Autodesk Inventor part; units mm, degrees
ref_plane "YZ Plane" through (0, 0, 0) normal (1, 0, 0) x (0, 1, 0)
ref_plane "XZ Plane" through (0, 0, 0) normal (0, 1, 0) x (-1, 0, 0)
ref_plane "XY Plane" through (0, 0, 0) normal (0, 0, 1) x (1, 0, 0)
sketch "Sketch1" plane through (0, 0, 0) normal (0, 1, 0) x (-1, 0, 0)
  line L0 (-25.4, 76.2) -> (25.4, 76.2)
  line L1 (50.8, 76.2) -> (-50.8, 76.2)
  line L2 (-50.8, 50.8) -> (-50.8, -50.8)
  line L3 (50.8, 76.2) -> (-50.8, 76.2)
  line L4 (-25.4, -76.2) -> (25.4, -76.2)
  line L5 (50.8, -50.8) -> (50.8, 50.8)
  arc A0 (50.8, 50.8) -> (25.4, 76.2) centre (25.4, 50.8) ccw
  arc A1 (25.4, -76.2) -> (50.8, -50.8) centre (25.4, -50.8) ccw
  arc A2 (-50.8, -50.8) -> (-25.4, -76.2) centre (-25.4, -50.8) ccw
  arc A3 (-25.4, 76.2) -> (-50.8, 50.8) centre (-25.4, 50.8) ccw
  circle A4 centre (-25.4, 50.8) radius 25.4
  circle A5 centre (-25.4, -50.8) radius 25.4
  circle A6 centre (-50.8, 0) radius 31.3961
  circle A7 centre (-82.1961, 0) radius 50.8
  circle A8 centre (25.4, -50.8) radius 2.5
  circle A9 centre (25.4, -50.8) radius 1.25
  circle A10 centre (25.4, 50.8) radius 2.5
  circle A11 centre (25.4, 50.8) radius 1.25
  circle A12 centre (-25.4, 50.8) radius 2.5
  circle A13 centre (-25.4, 50.8) radius 1.25
  circle A14 centre (-25.4, -50.8) radius 2.5
  circle A15 centre (-25.4, -50.8) radius 1.25
  line L6 (-31.3961, 0) -> (50.8, 0)
  point P0 (-36.7592, 28.0815)
  point P1 (-36.7592, -28.0815)
  point P2 (12.7, 38.1)
  point P3 (12.7, -38.1)
  point P4 (-50.8, -31.3961)
  point P5 (-50.8, 31.3961)
  point P6 (-44.332, -33.8667)
  point P7 (-44.332, 33.8667)
  point P8 (9.7019, 0)
  point P9 (0.3879, -59.1619)
  point P10 (-13.7063, -28.2519)
  dimension "d6" = 101.6
  dimension "d21" = 25.4
  dimension "d68" = 2.5
  dimension "d69" = 2.5
  dimension "d70" = 2.5
  dimension "d71" = 2.5
  dimension "d72" = 5
  dimension "d73" = 5
  dimension "d74" = 5
  dimension "d75" = 5
extrude "Extrusion4" add sketch "Sketch1" along normal blind 3 contours A4 A3 | L0 A0 L5 L6 A6 A4 | A4 A6 A7 | A6 L6 A7 | L5 A1 L4 A5 A6 L6 | A6 A7 L6 | A5 A2 | A7 A6 A5 | A8 | A9 | A10 | A11 | A12 | A13 | A14 | A15
hole "Hole3" at (-12.7, 0, 38.1) at (-12.7, 0, -38.1) direction (0, 1, 0) diameter 21 depth 25.4 tip angle 118
sketch "Sketch5" plane through (0, 0, 0) normal (0, -1, 0) x (1, 0, 0)
  arc A0 (36.7592, 28.0815) -> (36.7592, -28.0815) centre (50.8, 0) ccw
  arc A1 (36.7592, 28.0815) -> (36.7592, -28.0815) centre (50.8, 0) ccw
  arc A2 (44.332, 33.8667) -> (25.4, 76.2) centre (25.4, 50.8) ccw
  arc A3 (36.7592, 28.0815) -> (25.4, 76.2) centre (25.4, 50.8) ccw
  arc A4 (25.4, -76.2) -> (44.332, -33.8667) centre (25.4, -50.8) ccw
  arc A5 (25.4, -76.2) -> (36.7592, -28.0815) centre (25.4, -50.8) ccw
  arc A6 (-25.4, 76.2) -> (-50.8, 50.8) centre (-25.4, 50.8) ccw
  line L0 (-50.8, -50.8) -> (-50.8, 50.8)
  arc A7 (-25.4, 76.2) -> (-50.8, 50.8) centre (-25.4, 50.8) ccw
  arc A8 (-50.8, -50.8) -> (-25.4, -76.2) centre (-25.4, -50.8) ccw
  arc A9 (-50.8, -50.8) -> (-25.4, -76.2) centre (-25.4, -50.8) ccw
  line L1 (-25.4, 76.2) -> (25.4, 76.2)
  line L2 (25.4, 76.2) -> (-25.4, 76.2)
  line L3 (25.4, -76.2) -> (-25.4, -76.2)
  line L4 (25.4, -76.2) -> (-25.4, -76.2)
  line L5 (-50.8, 50.8) -> (-50.8, -50.8)
  arc A10 (44.332, 33.8667) -> (25.4, 76.2) centre (25.4, 50.8) ccw
  arc A11 (44.332, 33.8667) -> (44.332, -33.8667) centre (82.1961, 0) ccw
  arc A12 (44.332, 33.8667) -> (44.332, -33.8667) centre (82.1961, 0) ccw
  arc A13 (25.4, -76.2) -> (44.332, -33.8667) centre (25.4, -50.8) ccw
  arc A14 (-50.8, -50.8) -> (-25.4, -76.2) centre (-25.4, -50.8) ccw
  arc A15 (-25.4, 76.2) -> (-50.8, 50.8) centre (-25.4, 50.8) ccw
  arc A16 (-25.4, 76.2) -> (-50.8, 50.8) centre (-25.4, 50.8) ccw
  line L6 (-25.4, 76.2) -> (25.4, 76.2)
  line L7 (-50.8, 50.8) -> (-50.8, -50.8)
  line L8 (-25.4, -76.2) -> (25.4, -76.2)
  point P0 (0, 0)
  point P1 (-12.7, 38.1)
  point P2 (-12.7, -38.1)
extrude "Extrusion5" add sketch "Sketch5" along normal blind 30
shell "Shell1" thickness 3 removed faces 3 at (-23.4013, -30, 0) at (-13.5376, 0, 41.4983) at (-15.9531, 0, -34.6)
sketch "Sketch8" plane through (-50.8, 3, -50.8) normal (-1, 0, 0) x (0, 0, 1)
  line L0 (0, -33) -> (101.6, -33)
  line L1 (0, 0) -> (101.6, 0)
  line L2 (101.6, 0) -> (101.6, -33)
  line L3 (101.6, -33) -> (0, -33)
  line L4 (0, -33) -> (0, 0)
  line L5 (50.8, 0) -> (50.8, -33)
  line L6 (0, -16.5) -> (101.6, -16.5)
  line L7 (50.8, -16.5) -> (55.1, -16.5)
  line L8 (55.1, -16.5) -> (55.1, -14.7)
  line L9 (50.8, -16.5) -> (46.5, -16.5)
  line L10 (46.5, -16.5) -> (46.5, -18.3)
  line L11 (55.1, -14.7) -> (46.5, -14.7)
  line L12 (46.5, -14.7) -> (46.5, -18.3)
  line L13 (46.5, -18.3) -> (55.1, -18.3)
  line L14 (55.1, -18.3) -> (55.1, -14.7)
  point P0 (50.8, -3)
  dimension "d82" = 4.3
  dimension "d83" = 4.3
  dimension "d84" = 1.8
  dimension "d85" = 1.8
extrude "Extrusion8" cut sketch "Sketch8" against normal blind 2.54 contours L13 L10 L6 L5 | L5 L6 L14 L13 | L12 L11 L5 L6 | L5 L11 L8 L6
extrude "Extrusion9" add sketch "Sketch1" against normal blind 3 contours A8 | A10 | A12 | A14
equation "\"d69\" = d68"
equation "\"d70\" = d68"
equation "\"d71\" = d68"
equation "\"d73\" = d72"
equation "\"d74\" = d73"
equation "\"d75\" = d72"
equation "\"d83\" = d82"
equation "\"d85\" = d84"
properties part number "ControllerTop"
Part model, mm, in its own coordinate system. A direction names the side the tool comes from. Round coordinates to 2 decimals unless told otherwise and drop trailing zeros. Loops run counter-clockwise (first coordinate to the right, second up) from the corner with the lowest first, then second, coordinate; pieces in that order, holes last.
1. Two-plate mould, pull along X, no slides. Class faces 1 (the face through (31.4, 1.5, 0.5)), 2 (the face through (0, -15, 73.2)), 3 (the face through (-48.26, -13, 0)): pulls with the +X half, pulls with the -X half, needs draft (parallel to the pull), parting line crosses it, or undercut.
Solutions:
face 1: pulls with the +X half
face 2: undercut
face 3: pulls with the -X half
2. Slice it at A-A (x = -12.7). Give the cut face in (y, z).
Solutions:
outline: (-30, -76.2) - (3, -76.2) - (3, -48.6) - (0, -48.6) - (0, -73.2) - (-30, -73.2) - close; (-30, 73.2) - (0, 73.2) - (0, 48.6) - (3, 48.6) - (3, 76.2) - (-30, 76.2) - close; (0, -27.6) - (3, -27.6) - (3, 27.6) - (0, 27.6) - close
3. 3-axis set-ups, long thin cutter, end or side, ignore diameter. For faces 4 (the face through (-15.9, 1.5, -48.1)), 5 (the face through (28.4, -14.8, -0.5)): which of +Z, -Z, +X, -X, +Y, -Y reach the whole face in a straight line?
Solutions:
face 4: +Y, -Y
face 5: -Y
4. Slice it at C-C (z = -38.1). Give the cut face in (x, y).
Solutions:
outline: (-50.8, -30) - (-47.8, -30) - (-47.8, 0) - (-23.2, 0) - (-23.2, 3) - (-50.8, 3) - close; (-2.2, 0) - (43.85, 0) - (43.85, -30) - (47.4, -30) - (47.4, 3) - (-2.2, 3) - close
5. Slice it at B-B (y = -7). Give the cut face in (x, z), and give its area (3 significant figures).
Solutions:
outline: (-50.8, -50.8) arc R25.4 ccw to (-25.4, -76.2) - (25.4, -76.2) arc R25.4 ccw to (44.33, -33.87) arc R50.8 cw to (44.33, 33.87) arc R25.4 ccw to (25.4, 76.2) - (-25.4, 76.2) arc R25.4 ccw to (-50.8, 50.8) - close; hole (-47.8, -50.8) arc R22.4 ccw to (-25.4, -73.2) - (25.4, -73.2) arc R22.4 ccw to (42.1, -35.87) arc R53.8 cw to (42.1, 35.87) arc R22.4 ccw to (25.4, 73.2) - (-25.4, 73.2) arc R22.4 ccw to (-47.8, 50.8) - close
area: 1,390 mm2
6. Drill centre lines: line 1 along Z through (x, y) = (-2, -4); line 2 along Z through (x, y) = (25, -1); line 3 along Z through (x, y) = (43, -16). Where is each one in solid material? Low to high.
Solutions:
line 1: z = -76.2 to -73.2, 73.2 to 76.2
line 2: z = -76.2 to -73.2, -53.27 to -51.98, -49.62 to -48.33, 48.33 to 49.62, 51.98 to 53.27, 73.2 to 76.2
line 3: z = -69.11 to -64.66, -36.94 to -32.32, 32.32 to 36.94, 64.66 to 69.11
7. Flat gauge pins, fed straight in: pin 1 (19 mm diameter, centred on x = -12.7, z = -38.1, fed in from +Y); pin 2 (2.5 mm diameter, centred on x = 25, z = 51.5, fed in from -Y); pin 3 (0.8 mm diameter, centred on x = -25, z = -50.5, fed in from -Y); pin 4 (3 mm diameter, centred on y = -13.5, z = -1, fed in from -X). Where does each tip first touch, or does it go through?
Solutions:
pin 1: passes through
pin 2: stops at y = -3
pin 3: stops at y = 0
pin 4: stops at x = -48.26
8. Slice it at D-D (z = 1). Give the cut face in (x, y).
Solutions:
outline: (-50.8, -30) - (-47.8, -30) - (-47.8, 0) - (28.41, 0) - (28.41, -30) - (31.41, -30) - (31.41, 3) - (-50.8, 3) - (-50.8, -11.7) - (-48.26, -11.7) - (-48.26, -15.3) - (-50.8, -15.3) - close
